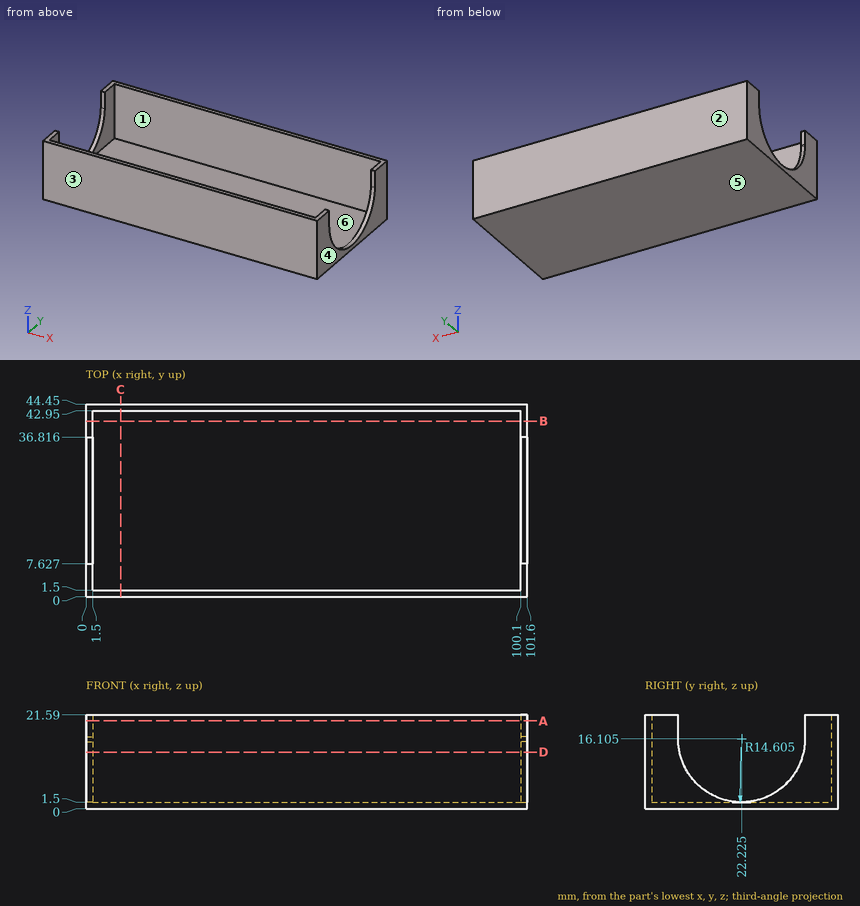
Can you work these out from the drawing? Everything is in mm from the part's minimum corner. A direction names the side the tool comes from. Give positions to 0.01 mm unless a question says otherwise; leave off trailing zeros. Order: outer loops, then holes, each group sorted by start corner. A loop starts at its lowest first (then second) coordinate and runs counter-clockwise, first axis right, second up.
Item 1: I need wall thicknesses on line 1 (Y direction, x = 67.5, z = 5.25); line 2 (X direction, y = 34.5, z = 2.5); line 3 (Z direction, x = 71.5, y = 8). Which ranges of each line are inside material? Lowest first, please.
Item 2: If we section it at A-A, the plane z = 20.25: Write out the boundary of the cut face in (x, y).
Item 3: If we section it at D-D, the plane z = 13: Write out the boundary of the cut face in (x, y).
Item 4: For the marked faces 5 and 6, which set-ups out of +Z, -Z, +X, -X, +Y, -Y let a thin tool reach every point of the face, with its end or its side?
Item 5: If we section it at B-B, the plane y = 40.5: Write out the boundary of the cut face in (x, z).
Item 6: If we mould it in two halves opening along Y, with no side actions, what happens to the marked faces 1, 2, 3 and 4? For each: pulls with the +Y half, pulls with the -Y half, needs draft (parallel to the pull), parting line crosses it, or undercut.
Item 7: If we section it at C-C, the plane x = 8: Write out the boundary of the cut face in (y, z), plus the area to 3 significant figures.
Item 8: I'm going to push a flat-ended pin straight in: pin 1 (1 mm diameter, centred on x = 55.5, y = 8.5, fed in from +Z). Where does the tip first touch, or does it pass through?
Values:
1. line 1: y = 0 to 1.5, 42.95 to 44.45
1. line 2: x = 0 to 1.5, 100.1 to 101.6
1. line 3: z = 0 to 1.5
2. outline: (0, 0) - (101.6, 0) - (101.6, 7.63) - (100.1, 7.63) - (100.1, 1.5) - (1.5, 1.5) - (1.5, 7.63) - (0, 7.63) - close; (0, 36.82) - (1.5, 36.82) - (1.5, 42.95) - (100.1, 42.95) - (100.1, 36.82) - (101.6, 36.82) - (101.6, 44.45) - (0, 44.45) - close
3. outline: (0, 0) - (101.6, 0) - (101.6, 7.95) - (100.1, 7.95) - (100.1, 1.5) - (1.5, 1.5) - (1.5, 7.95) - (0, 7.95) - close; (0, 36.5) - (1.5, 36.5) - (1.5, 42.95) - (100.1, 42.95) - (100.1, 36.5) - (101.6, 36.5) - (101.6, 44.45) - (0, 44.45) - close
4. face 5: -Z, +X, -X, +Y, -Y
4. face 6: +Z
5. outline: (0, 0) - (101.6, 0) - (101.6, 21.59) - (100.1, 21.59) - (100.1, 1.5) - (1.5, 1.5) - (1.5, 21.59) - (0, 21.59) - close
6. face 1: undercut
6. face 2: pulls with the +Y half
6. face 3: pulls with the -Y half
6. face 4: needs draft
7. outline: (0, 0) - (44.45, 0) - (44.45, 21.59) - (42.95, 21.59) - (42.95, 1.5) - (1.5, 1.5) - (1.5, 21.59) - (0, 21.59) - close
7. area: 127 mm2
8. pin 1: stops at z = 1.5
